```python
from build123d import *

# Parameters (mm, degrees)
F1_DEPTH      = 1524
F1_DEPTH_BACK = 25.4
F2_R          = 3.175
F3_DEPTH      = 38.1


with BuildPart() as f1:
    # F0 (on Front) → F1 (new body, two sides)
    with BuildSketch(Plane.XZ) as f1_sk:
        with BuildLine():
            Line((38.1, 38.1), (3.175, 38.1))
            ThreePointArc((3.175, 38.1), (0.929936, 37.170064), (0, 34.925))
            Line((0, 34.925), (0, 0))
            ThreePointArc((0, 0), (4.490128, 1.859872), (6.35, 6.35))
            Line((6.35, 6.35), (6.35, 25.4))
            ThreePointArc((6.35, 25.4), (8.209872, 29.890128), (12.7, 31.75))
            Line((12.7, 31.75), (31.75, 31.75))
            ThreePointArc((31.75, 31.75), (36.240128, 33.609872), (38.1, 38.1))
        make_face()
    extrude(amount=F1_DEPTH)
    extrude(f1_sk.sketch, amount=-F1_DEPTH_BACK)

    # F2 (on Right) → F3 (cut)
    with BuildSketch(Plane.YZ):
        with Locations((12.7, 9.525)):
            Circle(F2_R)
        with Locations((12.7, 22.225)):
            Circle(F2_R)
        with Locations((-1511.3, 9.525)):
            Circle(F2_R)
        with Locations((-1511.3, 22.225)):
            Circle(F2_R)
    extrude(amount=F3_DEPTH, mode=Mode.SUBTRACT)


solid = f1.part
```
Here's how the part is built. I have some questions about the finished solid (model axes, mm). Give positions to 0.01 mm unless a question says otherwise; leave off trailing zeros. Write each loop counter-clockwise with the first axis right and the second up, starting at its lowest first coordinate (ties: lowest second). Pieces come first, ordered by that corner, then holes. Notation, with made-up numbers: M 49.5,28.5 L 87.5,28.5 A28 ccw 87.5,64.5 Z; hole C 69.25,-31 d9. An arc over 180 degrees is marked long. Put each result on its own line as item: value. Start each with the question number.
Item 1: If we section it at A-A, the plane y = -1385.5: Write out the boundary of the cut face in (x, z) (3 decimals), then the cut area to 3 significant figures.
Item 2: I need wall thicknesses on L1, parallel to Z at x = 2.25, y = -1511.3; L2, parallel to Z at x = 4.25, y = -1511.3; L3, parallel to X at y = -752, z = 19. Which ranges of each line are inside material? Lowest first, please. Write a range as from..to.
Item 3: If we section it at B-B, the plane x = 24: Write out the boundary of the cut face in (y, z), then the cut area to 3 significant figures.
Item 4: Will these pins go through, and if not, where does the flat tip stop? pin 1 (1.5 mm diameter, centred on x = 14, y = -900.5, fed in from -Z); pin 2 (7.5 mm diameter, centred on y = -1511.3, z = 22.225, fed in from +X); pin 3 (1.5 mm diameter, centred on y = -346, z = 8, fed in from +X).
Values:
1. outline: M 0,0 A6.35 ccw 6.35,6.35 L 6.35,25.4 A6.35 cw 12.7,31.75 L 31.75,31.75 A6.35 ccw 38.1,38.1 L 3.175,38.1 A3.175 ccw 0,34.925 Z
1. area: 433 mm²
2. L1: 0.41..6.35, 12.7..19.05, 25.4..37.96
2. L2: 1.63..6.35, 12.7..19.05, 25.4..38.1
2. L3: 0..6.35
3. outline: M -1524,31.75 L 25.4,31.75 L 25.4,38.1 L -1524,38.1 Z
3. area: 9,840 mm²
4. pin 1: z = 31.75
4. pin 2: x = 6.38
4. pin 3: x = 6.35
